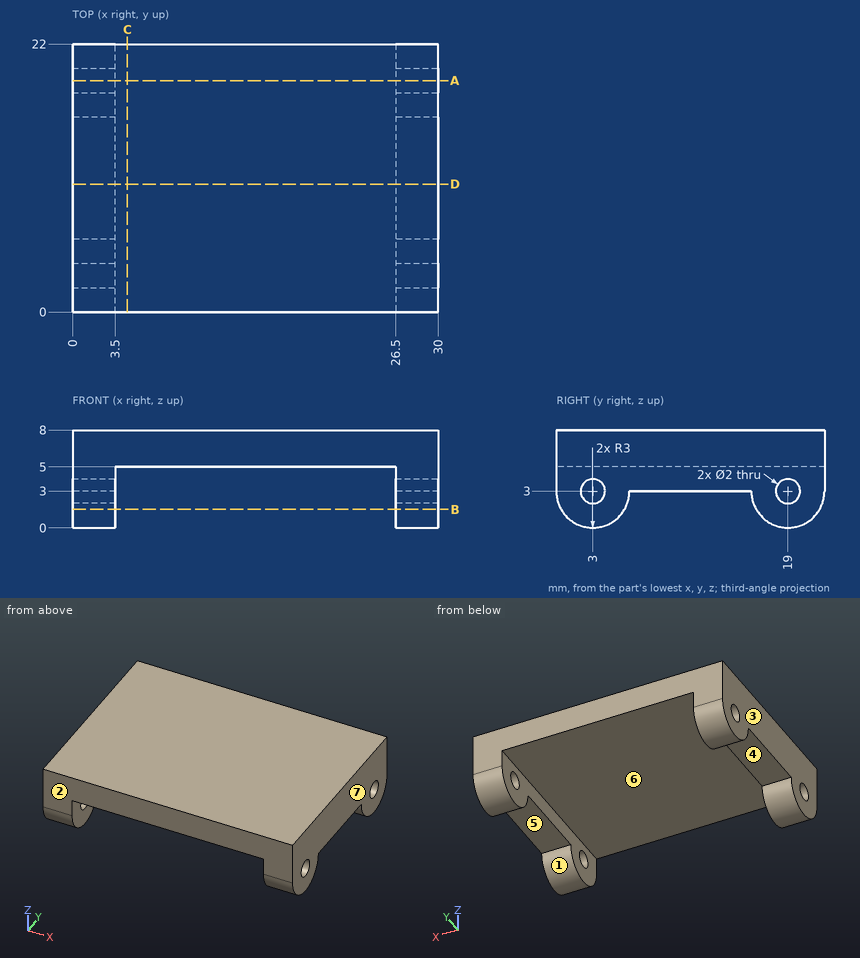
Here's the drawing with two shaded views (mm, measured from the low corner). I have some questions. A direction names the side the tool comes from. Coordinates: 2 decimals unless noted, no trailing zeros. Write each loop counter-clockwise with the first axis right and the second up, starting at its lowest first coordinate (ties: lowest second). Pieces come first, ordered by that corner, then holes. Notation, with made-up numbers: M 7,27 L 28,27 A10 ccw 28,34 Z; hole C 65.5,74.25 d11. An arc over 180 degrees is marked long. Answer as CSV lines item,"result". Start each with the question number.
1) Please list where these lines run through material, in increasing order: line 1 (X direction, y = 15, z = 3.75); line 2 (Z direction, x = 8.75, y = 10.25). Write a range as from..to.
2) I want a section at D-D, the plane y = 10.5. Please give me the cut outline in (x, z), and give its area (3 significant figures).
3) I want a section at B-B, the plane z = 1.5. Please give me the cut outline in (x, y), and give its area (3 significant figures).
4) For the marked faces 5, 6 and 7, which set-ups out of +Z, -Z, +X, -X, +Y, -Y let a thin tool reach every point of the face, with its end or its side?
5) I want a section at A-A, the plane y = 19. Please give me the cut outline in (x, z), and give its area (3 significant figures).
6) We'd pull the mould along Y, two halves only. Please class the marked faces 1, 2, 3 and 4: +Y half, -Y half, draft (parallel to the pull), parting line (faces both ways), or undercut.
7) I want a section at C-C, the plane x = 4.5. Please give me the cut outline in (y, z).
8) For P1, Ø1, axis at x = 28, y = 13.5, coming from the -Z side, with a flat end and sliding along its axis, tell me the tip position at first contact or that it passes through.
Data:
1,line 1,"x = 0..3.5, 26.5..30"
1,line 2,"z = 5..8"
2,outline,"M 0,3 L 3.5,3 L 3.5,5 L 26.5,5 L 26.5,3 L 30,3 L 30,8 L 0,8 Z"
2,area,"104 mm^2"
3,outline,"M 0,0.4 L 3.5,0.4 L 3.5,5.6 L 0,5.6 Z; M 0,16.4 L 3.5,16.4 L 3.5,21.6 L 0,21.6 Z; M 26.5,0.4 L 30,0.4 L 30,5.6 L 26.5,5.6 Z; M 26.5,16.4 L 30,16.4 L 30,21.6 L 26.5,21.6 Z"
3,area,"72.7 mm^2"
4,face 5,"-Z, +X, -X"
4,face 6,"-Z, +Y, -Y"
4,face 7,"+Z, -Z, +X, +Y, -Y"
5,outline,"M 0,0 L 3.5,0 L 3.5,2 L 0,2 Z; M 0,4 L 3.5,4 L 3.5,5 L 26.5,5 L 26.5,4 L 30,4 L 30,8 L 0,8 Z; M 26.5,0 L 30,0 L 30,2 L 26.5,2 Z"
5,area,"111 mm^2"
6,face 1,"undercut"
6,face 2,"-Y half"
6,face 3,"draft"
6,face 4,"undercut"
7,outline,"M 0,5 L 22,5 L 22,8 L 0,8 Z"
8,P1,"stops at z = 3"
